Geometry: final body of the model. Coordinates: model frame, mm. A direction names the side the tool comes from. Give positions to 0.01 mm unless a question says otherwise; leave off trailing zeros. Loops run counter-clockwise (first coordinate to the right, second up) from the corner with the lowest first, then second, coordinate; pieces in that order, holes last.
1. Section C-C, the plane y = 5. Output: boundary loops of the cut face in (x, z), then the cut area to 3 significant figures.
2. Section B-B, the plane x = -9. Output: boundary loops of the cut face in (y, z), then the cut area to 3 significant figures.
3. Section D-D, the plane y = 7.75. Output: boundary loops of the cut face in (x, z), then the cut area to 3 significant figures.
4. Draft query along Z for faces 1 (the face through (-9, 3.25, 2)), 2 (the face through (0, 6, 8)), 3 (the face through (0.35, 5.67, -0.99)). Return one class per face: +Z half, -Z half, draft (parallel to the pull), parting line (faces both ways), or undercut.
5. Section A-A, the plane z = 0. Output: boundary loops of the cut face in (x, y).
6. Material intervals for line 1 along Z through (x, y) = (-9, 2.2); line 2 along X through (y, z) = (6.25, 7.25); line 3 along X through (y, z) = (6, 3.5), sorted ascending.
7. Access query for faces 4 (the face through (-7.65, 1.6, 1.03)), 5 (the face through (-9, 4.75, 2)). Directions: +Z, -Z, +X, -X, +Y, -Y. A direction counts if a zero-diameter tool reaches every point of the face in a straight line with its end or side. Return the directions, or none.
from build123d import *

# Parameters (mm, degrees)
SKETCH1_W            = 23
SKETCH1_H            = 16
BOSS_EXTRUDE1_DEPTH  = 11.5
M6_CLEARANCE_HOLE3_D = 6.6
M3_CLEARANCE_HOLE1_D = 3.4
SKETCH9_R            = 1.55
CUT_EXTRUDE1_DEPTH   = 23.814469093
FILLET1_R            = 0.25


with BuildPart() as part:
    # Sketch1 → Boss-Extrude1 (new body)
    with BuildSketch(Plane(origin=(0, 0, 0), x_dir=(1, 0, 0), z_dir=(0, 1, 0))):
        Rectangle(SKETCH1_W, SKETCH1_H)
    extrude(amount=BOSS_EXTRUDE1_DEPTH)

    # M6 Clearance Hole3 (through all)
    with Locations(Plane(origin=(0, 11.5, 0), x_dir=(1, 0, 0), z_dir=(0, 1, 0))):
        with Locations((3.5, 0)):
            Hole(M6_CLEARANCE_HOLE3_D / 2)

    # M3 Clearance Hole1 (through all)
    with Locations(Plane(origin=(0, 11.5, 0), x_dir=(1, 0, 0), z_dir=(0, 1, 0))):
        with Locations((-9, 0), (9.5, 0)):
            Hole(M3_CLEARANCE_HOLE1_D / 2)

    # Sketch9 → Cut-Extrude1 (cut, through all)
    with BuildSketch(Plane.XY.offset(8)):
        with BuildLine():
            ThreePointArc((-5.90473751, 3.25), (-6, 4), (-5.90473751, 4.75))
            Line((-5.90473751, 4.75), (-11.5, 4.75))
            Line((-11.5, 4.75), (-11.5, 3.25))
            Line((-11.5, 3.25), (-5.90473751, 3.25))
        make_face()
        with BuildLine():
            ThreePointArc((0, 4), (-2.621987123, 6.976089089), (-5.90473751, 4.75))
            Line((-5.90473751, 4.75), (-5.90473751, 3.25))
            ThreePointArc((-5.90473751, 3.25), (-2.621987123, 1.023910911), (0, 4))
        make_face()
        with BuildLine():
            Line((-5.90473751, 3.25), (-5.90473751, 4.75))
            ThreePointArc((-5.90473751, 4.75), (-6, 4), (-5.90473751, 3.25))
        make_face()
        with Locations((9.5, 5.75)):
            Circle(SKETCH9_R)
    extrude(amount=-CUT_EXTRUDE1_DEPTH, mode=Mode.SUBTRACT)

    # Fillet1
    fillet1_edges = [part.edges().sort_by_distance(p)[0] for p in [
        (-11.5, 11.5, 0),
        (0, 11.5, 8),
        (-11.5, 1.625, 8),
        (-11.5, 1.625, -8),
        (11.5, 11.5, 0),
        (0, 0, 8),
        (-11.5, 0, 0),
        (0, 0, -8),
        (11.5, 0, 0),
        (0, 11.5, -8),
        (11.5, 5.75, 8),
        (-11.5, 8.125, 8),
        (-11.5, 8.125, -8),
        (11.5, 5.75, -8),
    ]]
    fillet(fillet1_edges, radius=FILLET1_R)


solid = part.part
Answers below:
1. outline: (-11.5, -7.75) arc R0.25 ccw to (-11.25, -8) - (-5.83, -8) - (-5.83, 8) - (-11.25, 8) arc R0.25 ccw to (-11.5, 7.75) - close; (-0.17, -8) - (8.14, -8) - (8.14, -1.02) arc R1.7 cw to (8.14, 1.02) - (8.14, 8) - (-0.17, 8) - close; (10.86, -8) - (11.25, -8) arc R0.25 ccw to (11.5, -7.75) - (11.5, 7.75) arc R0.25 ccw to (11.25, 8) - (10.86, 8) - (10.86, 1.02) arc R1.7 cw to (10.86, -1.02) - close; hole circle Ø3.4 at (-9, 0); hole circle Ø6.6 at (3.5, 0)
1. area: 190 mm2
2. outline: (0, -7.75) arc R0.25 ccw to (0.25, -8) - (3.25, -8) - (3.25, -1.7) - (0, -1.7) - close; (0, 1.7) - (3.25, 1.7) - (3.25, 8) - (0.25, 8) arc R0.25 ccw to (0, 7.75) - close; (4.75, -8) - (11.25, -8) arc R0.25 ccw to (11.5, -7.75) - (11.5, -1.7) - (4.75, -1.7) - close; (4.75, 1.7) - (11.5, 1.7) - (11.5, 7.75) arc R0.25 ccw to (11.25, 8) - (4.75, 8) - close
2. area: 126 mm2
3. outline: (-11.5, -7.75) arc R0.25 ccw to (-11.25, -8) - (11.25, -8) arc R0.25 ccw to (11.5, -7.75) - (11.5, 7.75) arc R0.25 ccw to (11.25, 8) - (-11.25, 8) arc R0.25 ccw to (-11.5, 7.75) - close; hole circle Ø3.4 at (-9, 0); hole circle Ø6.6 at (3.5, 0); hole circle Ø3.4 at (9.5, 0)
3. area: 316 mm2
4. face 1: draft
4. face 2: +Z half
4. face 3: undercut
5. outline: (-11.5, 0.25) arc R0.25 ccw to (-11.25, 0) - (-10.7, 0) - (-10.7, 3.25) - (-11.5, 3.25) - close; (-11.5, 4.75) - (-10.7, 4.75) - (-10.7, 11.5) - (-11.25, 11.5) arc R0.25 ccw to (-11.5, 11.25) - close; (-7.3, 0) - (0.2, 0) - (0.2, 11.5) - (-7.3, 11.5) - (-7.3, 4.75) - (-5.9, 4.75) arc R3 cw (long way) to (-5.9, 3.25) - (-7.3, 3.25) - close; (6.8, 0) - (7.8, 0) - (7.8, 11.5) - (6.8, 11.5) - close; (11.2, 0) - (11.25, 0) arc R0.25 ccw to (11.5, 0.25) - (11.5, 11.25) arc R0.25 ccw to (11.25, 11.5) - (11.2, 11.5) - close
6. line 1: z = -8 to -1.7, 1.7 to 8
6. line 2: x = -11.5 to -4.98, -1.02 to 8.03, 10.97 to 11.5
6. line 3: x = -11.5 to -5.24, -0.76 to 7.97, 11.03 to 11.5
7. face 4: +Y, -Y
7. face 5: +Z, -Z, -X
